For this review, take the finished solid that the model builds, in its own axes (mm). A direction names the side the tool comes from. Round coordinates to 2 decimals unless told otherwise and drop trailing zeros. Order: outer loops, then holes, each group sorted by start corner. A loop starts at its lowest first (then second) coordinate and runs counter-clockwise, first axis right, second up. Notation, with made-up numbers: M 42,5 L 92,5 A23 cw 92,15 Z; hole C 22.25,15 d6. An arc over 180 degrees is marked long. Answer as a JSON object with one key per item and string values.
from build123d import *

# Parameters (mm, degrees)
SKETCH1_R           = 170
BOSS_EXTRUDE1_DEPTH = 22.5
SKETCH2_R           = 170.69
BOSS_EXTRUDE2_DEPTH = 2
CUT_EXTRUDE3_START  = 10
SKETCH5_R           = 131.78
SKETCH5_R_2         = 60
CUT_EXTRUDE3_DEPTH  = 233.438450333
SKETCH6_R           = 30
CUT_EXTRUDE4_DEPTH  = 246.550712074
CUT_EXTRUDE5_DEPTH  = 246.550712074


with BuildPart() as part:
    # Sketch1 → Boss-Extrude1 (new, symmetric)
    with BuildSketch(Plane.XY):
        with Locations(Location((0, 0, 0), (0, 0, 180))):
            Circle(SKETCH1_R)
    extrude(amount=BOSS_EXTRUDE1_DEPTH, both=True)

    # Sketch2 → Boss-Extrude2 (add)
    with BuildSketch(Plane.XY.offset(22.5)):
        Circle(SKETCH2_R)
    boss_extrude2 = extrude(amount=-BOSS_EXTRUDE2_DEPTH)

    # Mirror1: Boss-Extrude2 across plane
    add(boss_extrude2.mirror(Plane.XY))

    # Sketch5 → Cut-Extrude3 (cut, through all)
    with BuildSketch(Plane.XY.offset(CUT_EXTRUDE3_START)):
        with Locations(Location((0, 0, 0), (0, 0, 180))):
            Circle(SKETCH5_R)
        with Locations(Location((0, 0, 0), (0, 0, 180))):
            Circle(SKETCH5_R_2, mode=Mode.SUBTRACT)
    cut_extrude3 = extrude(amount=CUT_EXTRUDE3_DEPTH, mode=Mode.SUBTRACT)

    # Mirror2: Cut-Extrude3 across plane
    add(cut_extrude3.mirror(Plane.XY), mode=Mode.SUBTRACT)

    # Sketch6 → Cut-Extrude4 (cut, through all)
    with BuildSketch(Plane.XY.offset(22.5)):
        Circle(SKETCH6_R)
    extrude(amount=-CUT_EXTRUDE4_DEPTH, mode=Mode.SUBTRACT)

    # Sketch7 → Cut-Extrude5 (cut, through all)
    with BuildSketch(Plane.XY.offset(22.5)):
        with BuildLine():
            Line((9, 20.2728873), (9, 34.650252524))
            ThreePointArc((9, 34.650252524), (0, 35.8), (-9, 34.650252524))
            Line((-9, 34.650252524), (-9, 20.2728873))
            Line((-9, 20.2728873), (9, 20.2728873))
        make_face()
    extrude(amount=-CUT_EXTRUDE5_DEPTH, mode=Mode.SUBTRACT)


solid = part.part
1) Insertion check: P1, Ø4, axis at y = 49, z = -18, coming from the +X side; P2, Ø2, axis at x = 97.5, y = 73, coming from the -Z side; P3, Ø12, axis at y = 71, z = 13.5, coming from the +X side. Each pin has a flat end and moves straight along its axis. Give the tip position at first contact, or say it passes through.
Geometry check:
{"P1": "stops at x = 163.37", "P2": "stops at z = -10", "P3": "stops at x = 157.08"}
2) Add section A-A on z = -15. State the section outline as (x, y) points, and give its area (3 significant figures).
Geometry check:
{"outline": "C 0,0 d340; C 0,0 d120; hole C 0,0 d263.56; hole M -9,28.62 A30 ccw long 9,28.62 L 9,34.65 A35.8 ccw -9,34.65 Z", "area": "44,600 mm²"}
3) Add section D-D on y = -146.5. State the section outline as (x, z) points.
Geometry check:
{"outline": "M -87.59,-22.5 L 87.59,-22.5 L 87.59,-20.5 L 86.24,-20.5 L 86.24,20.5 L 87.59,20.5 L 87.59,22.5 L -87.59,22.5 L -87.59,20.5 L -86.24,20.5 L -86.24,-20.5 L -87.59,-20.5 Z"}
4) Machinability: for faces 1 (the flat face through (12, 28, 22.5)), 2 (the flat face through (88, -100, -22.5)), 3 (the cylindrical face through (0.1, 35.8, 0.3)), 4 (the cylindrical face through (131.653, -5.794, 16.163)), 5 (the cylindrical face through (131.653, -5.794, -16.163)), which of the approach directions +Z, -Z, +X, -X, +Y, -Y give a long, thin tool a straight path to every point of the face, cutting with its end or side? Answer none if there is none.
Geometry check:
{"face 1": "+Z, +X, -X, +Y, -Y", "face 2": "-Z, +X, -X, +Y, -Y", "face 3": "+Z, -Z", "face 4": "+Z", "face 5": "-Z"}
5) Mouldability with a two-part tool opening along Z and no side actions: class faces 6 (the cylindrical face through (-162.15, -51.06, 0.29)), 7 (the cylindrical face through (-32.26, -50.59, 16.16)), 8 (the flat face through (-27, 57, 10)) as +Z half, -Z half, draft (parallel to the pull), parting line (faces both ways), or undercut.
Geometry check:
{"face 6": "undercut", "face 7": "draft", "face 8": "+Z half"}
6) For L1, parallel to Y at x = 0, z = 15.25; L2, parallel to Y at x = 0, z = 1.5; L3, parallel to Y at x = -17, z = -14.5, list the stretches that pass through material, from the lowest coordinate up.
Geometry check:
{"L1": "y = -170 to -131.78, -60 to -30, 35.8 to 60, 131.78 to 170", "L2": "y = -170 to -30, 35.8 to 170", "L3": "y = -169.15 to -130.68, -57.54 to -24.72, 24.72 to 57.54, 130.68 to 169.15"}
